```python
from build123d import *

# Parameters (mm, degrees)
ESQUISSE1_R        = 0.381
ESQUISSE1_R_2      = 2.839806331
ESQUISSE1_R_3      = 0.5
BOSS_EXTRU_1_DEPTH = 1.6


with BuildPart() as part:
    # Esquisse1 → Boss.-Extru.1 (new body)
    with BuildSketch(Plane.XY.offset(1.6)):
        with BuildLine():
            Line((146.05, -111.76), (146.05, -57.15))
            ThreePointArc((146.05, -57.15), (144.934076836, -54.455923164), (142.24, -53.34))
            Line((142.24, -53.34), (27.94, -53.34))
            ThreePointArc((27.94, -53.34), (25.245923164, -54.455923164), (24.13, -57.15))
            Line((24.13, -57.15), (24.13, -111.76))
            ThreePointArc((24.13, -111.76), (25.245923164, -114.454076836), (27.94, -115.57))
            Line((27.94, -115.57), (142.24, -115.57))
            ThreePointArc((142.24, -115.57), (144.934076836, -114.454076836), (146.05, -111.76))
        make_face()
        with Locations((55.88, -109.22)):
            Circle(ESQUISSE1_R, mode=Mode.SUBTRACT)
        with Locations((55.88, -106.68)):
            Circle(ESQUISSE1_R, mode=Mode.SUBTRACT)
        with Locations((142.24, -111.76)):
            Circle(ESQUISSE1_R_2, mode=Mode.SUBTRACT)
        with Locations((81.28, -111.76)):
            Circle(ESQUISSE1_R_2, mode=Mode.SUBTRACT)
        with Locations((76.2, -106.68)):
            Circle(ESQUISSE1_R, mode=Mode.SUBTRACT)
        with Locations((76.2, -109.22)):
            Circle(ESQUISSE1_R, mode=Mode.SUBTRACT)
        with Locations((76.2, -104.14)):
            Circle(ESQUISSE1_R, mode=Mode.SUBTRACT)
        with Locations((55.88, -104.14)):
            Circle(ESQUISSE1_R, mode=Mode.SUBTRACT)
        with Locations((142.24, -58.42)):
            Circle(ESQUISSE1_R_3, mode=Mode.SUBTRACT)
        with Locations((142.24, -69.85)):
            Circle(ESQUISSE1_R_2, mode=Mode.SUBTRACT)
        with Locations((142.24, -60.96)):
            Circle(ESQUISSE1_R_3, mode=Mode.SUBTRACT)
        with Locations((142.24, -63.5)):
            Circle(ESQUISSE1_R_3, mode=Mode.SUBTRACT)
        with Locations((80.01, -63.5)):
            Circle(ESQUISSE1_R_2, mode=Mode.SUBTRACT)
        with Locations((55.88, -71.12)):
            Circle(ESQUISSE1_R, mode=Mode.SUBTRACT)
        with Locations((55.88, -73.66)):
            Circle(ESQUISSE1_R, mode=Mode.SUBTRACT)
        with Locations((55.88, -76.2)):
            Circle(ESQUISSE1_R, mode=Mode.SUBTRACT)
        with Locations((55.88, -78.74)):
            Circle(ESQUISSE1_R, mode=Mode.SUBTRACT)
        with Locations((42.672, -66.04)):
            Circle(ESQUISSE1_R, mode=Mode.SUBTRACT)
        with Locations((35.052, -66.04)):
            Circle(ESQUISSE1_R, mode=Mode.SUBTRACT)
        with Locations((37.592, -66.04)):
            Circle(ESQUISSE1_R, mode=Mode.SUBTRACT)
        with Locations((40.132, -66.04)):
            Circle(ESQUISSE1_R, mode=Mode.SUBTRACT)
        with Locations((76.2, -81.28)):
            Circle(ESQUISSE1_R, mode=Mode.SUBTRACT)
        with Locations((55.88, -81.28)):
            Circle(ESQUISSE1_R, mode=Mode.SUBTRACT)
        with Locations((76.2, -83.82)):
            Circle(ESQUISSE1_R, mode=Mode.SUBTRACT)
        with Locations((76.2, -86.36)):
            Circle(ESQUISSE1_R, mode=Mode.SUBTRACT)
        with Locations((76.2, -88.9)):
            Circle(ESQUISSE1_R, mode=Mode.SUBTRACT)
        with Locations((55.88, -86.36)):
            Circle(ESQUISSE1_R, mode=Mode.SUBTRACT)
        with Locations((55.88, -88.9)):
            Circle(ESQUISSE1_R, mode=Mode.SUBTRACT)
        with Locations((55.88, -83.82)):
            Circle(ESQUISSE1_R, mode=Mode.SUBTRACT)
        with Locations((76.2, -93.98)):
            Circle(ESQUISSE1_R, mode=Mode.SUBTRACT)
        with Locations((55.88, -93.98)):
            Circle(ESQUISSE1_R, mode=Mode.SUBTRACT)
        with Locations((76.2, -91.44)):
            Circle(ESQUISSE1_R, mode=Mode.SUBTRACT)
        with Locations((55.88, -91.44)):
            Circle(ESQUISSE1_R, mode=Mode.SUBTRACT)
        with Locations((76.2, -96.52)):
            Circle(ESQUISSE1_R, mode=Mode.SUBTRACT)
        with Locations((76.2, -99.06)):
            Circle(ESQUISSE1_R, mode=Mode.SUBTRACT)
        with Locations((76.2, -101.6)):
            Circle(ESQUISSE1_R, mode=Mode.SUBTRACT)
        with Locations((55.88, -101.6)):
            Circle(ESQUISSE1_R, mode=Mode.SUBTRACT)
        with Locations((55.88, -99.06)):
            Circle(ESQUISSE1_R, mode=Mode.SUBTRACT)
        with Locations((55.88, -96.52)):
            Circle(ESQUISSE1_R, mode=Mode.SUBTRACT)
        with BuildLine():
            Line((32.925, -63.747), (30.925, -63.747))
            ThreePointArc((30.925, -63.747), (30.425, -63.247), (30.925, -62.747))
            Line((30.925, -62.747), (32.925, -62.747))
            ThreePointArc((32.925, -62.747), (33.425, -63.247), (32.925, -63.747))
        make_face(mode=Mode.SUBTRACT)
        with BuildLine():
            Line((29.425, -57.547), (29.425, -59.547))
            ThreePointArc((29.425, -59.547), (28.925, -60.047), (28.425, -59.547))
            Line((28.425, -59.547), (28.425, -57.547))
            ThreePointArc((28.425, -57.547), (28.925, -57.047), (29.425, -57.547))
        make_face(mode=Mode.SUBTRACT)
        with BuildLine():
            Line((35.425, -57.547), (35.425, -59.547))
            ThreePointArc((35.425, -59.547), (34.925, -60.047), (34.425, -59.547))
            Line((34.425, -59.547), (34.425, -57.547))
            ThreePointArc((34.425, -57.547), (34.925, -57.047), (35.425, -57.547))
        make_face(mode=Mode.SUBTRACT)
    extrude(amount=-BOSS_EXTRU_1_DEPTH)


solid = part.part
```
Check sheet for the modelled part. Datum: model origin and axes. Units: mm. Give positions to 0.01 mm unless a question says otherwise; leave off trailing zeros. Answer in a Markdown table with one row per item. Add a question column.
Q1. Gauge pin test, flat end, axial feed: pin 1 Ø2 at (x, y) = (113.5, -92.5) entering from -Z. Record the tip position at first contact, or that the pin passes through.
Q2. Sectioned sample at A-A, the plane z = 0.25. Count the separate pieces of the cut face and the enclosed holes in it, and give its area (3 significant figures).
Q3. Release check for a two-part mould opening along Y. For faces 1 (the cylindrical face through (144.95, -110.91, 0.81)), 2 (the cylindrical face through (25.276, -54.426, 0.811)), 3 (the cylindrical face through (144.904, -114.484, 0.811)) record: released by +Y, released by -Y, zero draft, split by the parting line, or undercut.
Q4. Thickness scan on L1, parallel to X at y = -89, z = 1.4; L2, parallel to X at y = -91.44, z = 1.2; L3, parallel to Y at x = 79.5, z = 1.25. Record the ranges inside material, lowest first.
Verdict:
| question | item | result |
|---|---|---|
| 1 | pin 1 | z = 0 |
| 2 | separate pieces | 1 |
| 2 | enclosed holes | 42 |
| 2 | area | 7,450 mm² |
| 3 | face 1 | undercut |
| 3 | face 2 | released by +Y |
| 3 | face 3 | released by -Y |
| 4 | L1 | 24.13 to 55.51, 56.25 to 75.83, 76.57 to 146.05 |
| 4 | L2 | 24.13 to 55.5, 56.26 to 75.82, 76.58 to 146.05 |
| 4 | L3 | -115.57 to -113.97, -109.55 to -66.29, -60.71 to -53.34 |
